from build123d import *

# Parameters (mm, degrees)
SKETCH_1_W            = 381
SKETCH_1_H            = 181
EXTRUDE_1_DEPTH       = 25
CUT_EXTRUDE_1_DEPTH   = 25
EXTRUDE_START         = 4
EXTRUDE_2_DEPTH       = 4
MIRROR_2_COPY_1_DEPTH = 25
MIRROR_START          = 4
MIRROR_2_COPY_2_DEPTH = 4
MIRROR_2_COPY_3_DEPTH = 25


with BuildPart() as part:
    # Sketch 1 → Extrude 1 (new body)
    with BuildSketch(Plane(origin=(0, 0, 0), x_dir=(1, 0, 0), z_dir=(0, 1, 0))):
        Rectangle(SKETCH_1_W, SKETCH_1_H)
    extrude(amount=EXTRUDE_1_DEPTH)

    # Sketch 2 → Cut-Extrude 1 (cut)
    with BuildSketch(Plane(origin=(0, 25, 0), x_dir=(1, 0, 0), z_dir=(0, 1, 0))):
        with BuildLine():
            Line((-190.5, 57.5), (-170.5, 57.5))
            ThreePointArc((-170.5, 57.5), (-163.5, 64.5), (-170.5, 71.5))
            Line((-170.5, 71.5), (-190.5, 71.5))
            Line((-190.5, 71.5), (-190.5, 57.5))
        make_face()
    cut_extrude_1 = extrude(amount=-CUT_EXTRUDE_1_DEPTH, mode=Mode.SUBTRACT)

    # Sketch 2_3 → Extrude 2 (add)
    with BuildSketch(Plane(origin=(0, 25, 0), x_dir=(1, 0, 0), z_dir=(0, 1, 0)).offset(EXTRUDE_START)):
        with BuildLine():
            ThreePointArc((-170.5, 71.5), (-163.5, 64.5), (-170.5, 57.5))
            Line((-170.5, 57.5), (-190.5, 57.5))
            Line((-190.5, 57.5), (-190.5, 49.5))
            Line((-190.5, 49.5), (-170.5, 49.5))
            ThreePointArc((-170.5, 49.5), (-155.5, 64.5), (-170.5, 79.5))
            Line((-170.5, 79.5), (-190.5, 79.5))
            Line((-190.5, 79.5), (-190.5, 71.5))
            Line((-190.5, 71.5), (-170.5, 71.5))
        make_face()
    extrude_2 = extrude(amount=-EXTRUDE_2_DEPTH)

    # Mirror 1: Cut-Extrude 1, Extrude 2 across plane
    add(cut_extrude_1.mirror(Plane.XY), mode=Mode.SUBTRACT)
    add(extrude_2.mirror(Plane.XY))

    # Mirror 2: Extrude 2 across plane
    add(extrude_2.mirror(Plane(origin=(0, 0, 0), x_dir=(0, 0, 1), z_dir=(1, 0, 0))))

    # Mirror 2 copy 1 sketch → Mirror 2 copy 1 (cut)
    with BuildSketch(Plane(origin=(0, 25, 0), x_dir=(-1, 0, 0), z_dir=(0, 1, 0))):
        with BuildLine():
            Line((-190.5, 57.5), (-170.5, 57.5))
            ThreePointArc((-170.5, 57.5), (-163.5, 64.5), (-170.5, 71.5))
            Line((-170.5, 71.5), (-190.5, 71.5))
            Line((-190.5, 71.5), (-190.5, 57.5))
        make_face()
    extrude(amount=-MIRROR_2_COPY_1_DEPTH, mode=Mode.SUBTRACT)

    # Mirror 2 copy 2 sketch → Mirror 2 copy 2 (add)
    with BuildSketch(Plane(origin=(0, 25, 0), x_dir=(-1, 0, 0), z_dir=(0, 1, 0)).offset(MIRROR_START)):
        with BuildLine():
            ThreePointArc((-170.5, 71.5), (-163.5, 64.5), (-170.5, 57.5))
            Line((-170.5, 57.5), (-190.5, 57.5))
            Line((-190.5, 57.5), (-190.5, 49.5))
            Line((-190.5, 49.5), (-170.5, 49.5))
            ThreePointArc((-170.5, 49.5), (-155.5, 64.5), (-170.5, 79.5))
            Line((-170.5, 79.5), (-190.5, 79.5))
            Line((-190.5, 79.5), (-190.5, 71.5))
            Line((-190.5, 71.5), (-170.5, 71.5))
        make_face()
    extrude(amount=-MIRROR_2_COPY_2_DEPTH)

    # Mirror 2 copy 3 sketch → Mirror 2 copy 3 (cut)
    with BuildSketch(Plane(origin=(0, 25, 0), x_dir=(-1, 0, 0), z_dir=(0, 1, 0))):
        with BuildLine():
            Line((-190.5, -57.5), (-170.5, -57.5))
            ThreePointArc((-170.5, -57.5), (-163.5, -64.5), (-170.5, -71.5))
            Line((-170.5, -71.5), (-190.5, -71.5))
            Line((-190.5, -71.5), (-190.5, -57.5))
        make_face()
    extrude(amount=-MIRROR_2_COPY_3_DEPTH, mode=Mode.SUBTRACT)


solid = part.part
The listing builds one solid part. Answer for the finished solid, in the listing's coordinates (mm). A direction names the side the tool comes from. Give positions to 0.01 mm unless a question says otherwise; leave off trailing zeros. Write each loop counter-clockwise with the first axis right and the second up, starting at its lowest first coordinate (ties: lowest second). Pieces come first, ordered by that corner, then holes.
1) Section B-B (y = 8.5) is taken. Write down the section's boundary in (x, z).
2) Given P1, Ø1.5, axis at y = 18, z = -68.5, coming from the -X side; P2, Ø3, axis at x = 185, y = 27, coming from the +Z side; P3, Ø8, axis at y = 18, z = -66.5, coming from the +X side, each flat-ended and moving along its own axis, determine where each tip first touches the part or whether it passes through.
3) For a pull along X with two mould halves and no side action, classify faces 4 (the face through (180, 15, -71.5)), 5 (the face through (-155.504, 27.028, 64.17)), 6 (the face through (190.5, 15, 81)) as pulls with the +X half, pulls with the -X half, needs draft (parallel to the pull), parting line crosses it, or undercut.
4) Section C-C (x = 9) is taken. Write down the section's boundary in (y, z), and give its area (4 significant figures).
5) A tool of negligible diameter and unlimited length cuts with its end or side. For faces 1 (the face through (-155.504, 27.028, -64.17)), 2 (the face through (180, 15, 57.5)), 3 (the face through (-180, 15, -57.5)), from which of +Z, -Z, +X, -X, +Y, -Y can it reach the whole face along a straight path? Write none if from no direction.
6) Section A-A (z = 64.5) is taken. Write down the section's boundary in (x, y), and give its area (3 significant figures).
7) Find the intervals of material crossed by L1, parallel to Y at x = 93.5, z = 42; L2, parallel to X at y = 2, z = -60; L3, parallel to X at y = 7, z = -62.5, in increasing order.
8) Section D-D (z = 37.5) is taken. Write down the section's boundary in (x, y), and give its area (4 significant figures).
Response:
1. outline: (-190.5, -90.5) - (190.5, -90.5) - (190.5, -71.5) - (170.5, -71.5) arc R7 cw to (170.5, -57.5) - (190.5, -57.5) - (190.5, 57.5) - (170.5, 57.5) arc R7 cw to (170.5, 71.5) - (190.5, 71.5) - (190.5, 90.5) - (-190.5, 90.5) - (-190.5, 71.5) - (-170.5, 71.5) arc R7 cw to (-170.5, 57.5) - (-190.5, 57.5) - (-190.5, -57.5) - (-170.5, -57.5) arc R7 cw to (-170.5, -71.5) - (-190.5, -71.5) - close
2. P1: stops at x = -165.36
2. P2: stops at z = 79.5
2. P3: stops at x = 166.89
3. face 4: needs draft
3. face 5: undercut
3. face 6: pulls with the +X half
4. outline: (0, -90.5) - (25, -90.5) - (25, 90.5) - (0, 90.5) - close
4. area: 4,525 mm2
5. face 1: +Y
5. face 2: +X, +Y, -Y
5. face 3: -X, +Y, -Y
6. outline: (-163.5, 0) - (163.5, 0) - (163.5, 29) - (155.5, 29) - (155.5, 25) - (-155.5, 25) - (-155.5, 29) - (-163.5, 29) - close
6. area: 8,240 mm2
7. L1: y = 0 to 25
7. L2: x = -165.14 to 165.14
7. L3: x = -163.79 to 163.79
8. outline: (-190.5, 0) - (190.5, 0) - (190.5, 25) - (-190.5, 25) - close
8. area: 9,525 mm2
